Read the model definition and answer for the solid it produces. Units are mm, in the model's axes. Face numbers are marked on the shaded views. Round coordinates to 2 decimals unless told otherwise and drop trailing zeros. Order: outer loops, then holes, each group sorted by start corner. A loop starts at its lowest first (then second) coordinate and runs counter-clockwise, first axis right, second up. Notation, with made-up numbers: (79.25, 54.5) -> (113.25, 54.5) arc R26 ccw to (113.25, 80.5) -> close; hole circle Ø7 at (-4.5, 45.5). An arc over 180 degrees is marked (long way). Use a Markdown table: item, result. Add a question column.
1. The mould has two halves that part along Z. Classify the marked faces 1, 2, 3 and 4: +Z half, -Z half, draft (parallel to the pull), parting line (faces both ways), or undercut.
2. Consider L1, parallel to Z at x = -42.5, y = -8.25; L2, parallel to X at y = -5.25, z = -8; L3, parallel to Z at x = -19.5, y = -14.5. Determine where each line is inside the solid, lowest interval first. Write a range as [from, to].
3. Section B-B, the plane x = -49 is taken. Give the vertices of the cut face in (y, z), then the cut area to 3 significant figures.
4. Section C-C, the plane y = -14.75 is taken. Give the vertices of the cut face in (x, z).
5. Section A-A, the plane z = 29 is taken. Give the vertices of the cut face in (x, y), then the cut area to 3 significant figures.
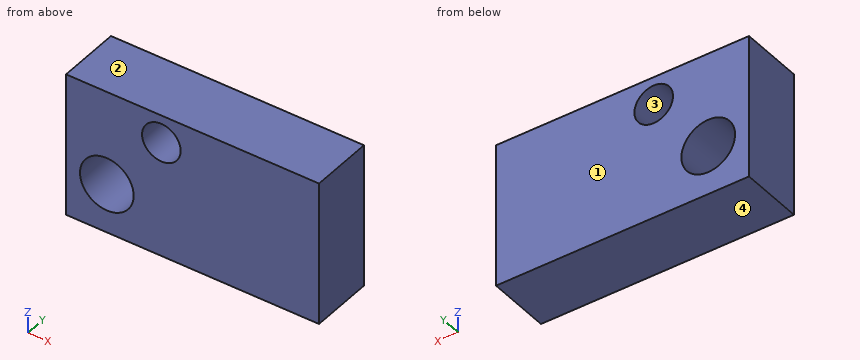
```python
from build123d import *

# Parameters (mm, degrees)
F0_W     = 100.13302
F0_H     = 56.984361
F1_DEPTH = 25
F2_R     = 7.642085
F3_DEPTH = 120.5
F4_R     = 10.630728
F5_DEPTH = 179


with BuildPart() as f1:
    # F0 (on Front) → F1 (new body)
    with BuildSketch(Plane.XZ):
        with Locations((-9.035291, 6.027846)):
            Rectangle(F0_W, F0_H)
    extrude(amount=F1_DEPTH)

    # F2 (on Front) → F3 (cut)
    with BuildSketch(Plane.XZ):
        with Locations((-21.377444, 23.498362)):
            Circle(F2_R)
    extrude(amount=F3_DEPTH, mode=Mode.SUBTRACT)

    # F4 (on Front) → F5 (cut)
    with BuildSketch(Plane.XZ):
        with Locations((-42.96153, -2.936909)):
            Circle(F4_R)
    extrude(amount=F5_DEPTH, mode=Mode.SUBTRACT)


solid = f1.part
```
Verdict:
| question | item | result |
|---|---|---|
| 1 | face 1 | draft |
| 1 | face 2 | +Z half |
| 1 | face 3 | undercut |
| 1 | face 4 | -Z half |
| 2 | L1 | z = [-22.46, -13.56], [7.68, 34.52] |
| 2 | L2 | x = [-59.1, -52.31], [-33.61, 41.03] |
| 2 | L3 | z = [-22.46, 16.09], [30.91, 34.52] |
| 3 | outline | (-25, -22.46) -> (0, -22.46) -> (0, -11.69) -> (-25, -11.69) -> close; (-25, 5.81) -> (0, 5.81) -> (0, 34.52) -> (-25, 34.52) -> close |
| 3 | area | 987 mm2 |
| 4 | outline | (-59.1, -22.46) -> (41.03, -22.46) -> (41.03, 34.52) -> (-59.1, 34.52) -> close; hole circle Ø21.26 at (-42.96, -2.94); hole circle Ø15.28 at (-21.38, 23.5) |
| 5 | outline | (-59.1, -25) -> (-26.68, -25) -> (-26.68, 0) -> (-59.1, 0) -> close; (-16.07, -25) -> (41.03, -25) -> (41.03, 0) -> (-16.07, 0) -> close |
| 5 | area | 2,240 mm2 |
